```python
from build123d import *

# Parameters (mm, degrees)
F1_W          = 3
F1_H          = 12
F2_DEPTH      = 5
F2_DEPTH_BACK = 5
F4_R          = 3
F5_R          = 2.99999
F7_DEPTH      = 25
F8_R          = 3


# Not quite as in the source:
# - a fillet or chamfer is up to 0.001 mm smaller than in the source, because OpenCascade refuses the exact size


with BuildPart() as f2:
    # F1 (on Front) → F2 (new body, two sides)
    with BuildSketch(Plane.XZ) as f2_sk:
        with Locations((-19, -6)):
            Rectangle(F1_W, F1_H)
        Polygon((-20.5, 0), (-17.5, 0), (-17.5, 12), (-23.5, 12), (-23.5, -22), (-36.5, -22), (-36.5, -25), (-20.5, -25), (-20.5, -12), align=None)
    extrude(amount=F2_DEPTH)
    extrude(f2_sk.sketch, amount=-F2_DEPTH_BACK)

    # F0 (on Front) → F3 (revolve, cut)
    with BuildSketch(Plane.XZ):
        with BuildLine():
            Line((0, -20.5), (0, 20.5))
            ThreePointArc((0, 20.5), (-20.5, 0), (0, -20.5))
        make_face()
    revolve(axis=Axis((0, 0, 0), (0, 0, 1)), mode=Mode.SUBTRACT)

    # F4
    f4_edges = [f2.edges().sort_by_distance(p)[0] for p in [
        (-23.5, 0, 12),
        (-23.5, 0, -22),
    ]]
    fillet(f4_edges, radius=F4_R)

    # F5 (radius 3 in the source; OpenCascade refuses exactly that, so slightly less here)
    f5_edges = [f2.edges().sort_by_distance(p)[0] for p in [
        (-20.5, 0, -12),
    ]]
    fillet(f5_edges, radius=F5_R)

    # F6 (on face) → F7 (cut)
    with BuildSketch(Plane.XY.offset(-22)):
        with BuildLine():
            ThreePointArc((-29.75, 0), (-30.8303039934, 1.6167891819), (-32.7374368671, 1.2374368671))
            Line((-32.7374368671, 1.2374368671), (-30.2625631329, -1.2374368671))
            ThreePointArc((-30.2625631329, -1.2374368671), (-29.8832108181, -0.6696960066), (-29.75, 0))
        make_face()
        with BuildLine():
            Line((-30.2625631329, -1.2374368671), (-32.7374368671, 1.2374368671))
            ThreePointArc((-32.7374368671, 1.2374368671), (-32.7374368671, -1.2374368671), (-30.2625631329, -1.2374368671))
        make_face()
    extrude(amount=-F7_DEPTH, mode=Mode.SUBTRACT)

    # F8
    f8_edges = [f2.edges().sort_by_distance(p)[0] for p in [
        (-36.5, -5, -23.5),
        (-36.5, 5, -23.5),
    ]]
    fillet(f8_edges, radius=F8_R)


solid = f2.part
```
Verification items for the finished model (mm, model axes). A direction names the side the tool comes from. Coordinates: 2 decimals unless noted, no trailing zeros. Order: outer loops, then holes, each group sorted by start corner. A loop starts at its lowest first (then second) coordinate and runs counter-clockwise, first axis right, second up. Notation, with made-up numbers: (88.5, -25) -> (130.5, -25) arc R24 cw to (130.5, 13) -> close; hole circle Ø10 at (83, 12). An arc over 180 degrees is marked (long way). Put each result on its own line as item: value. Start each with the question number.
1) Tool access check on faces 1 (the flat face through (-20.5, 0, -20)), 2 (the flat face through (-23, 5, -8)), 3 (the flat face through (-29, 0, -22)). Record the directions out of +Z, -Z, +X, -X, +Y, -Y that give a thin tool (end or side, any length) a straight path to the whole face; none if there is none.
2) Cross-section at D-D (x = -27.75). Enter the section's corners in (y, z), plus the area to 3 significant figures.
3) Material ranges on L1, parallel to X at y = -1.5, z = -18; L2, parallel to Z at x = -33, y = 4; L3, parallel to Z at x = -24, y = -0.75, recorded low to high.
4) Cross-section at A-A (x = -31.5). Enter the section's corners in (y, z).
5) Cross-section at C-C (z = -18). Enter the section's corners in (x, y), plus the area to 3 significant figures.
6) Go/stop test with flat-tipped pins: pin 1 (5 mm diameter, centred on y = -1, z = -2.5, fed in from +X); pin 2 (4 mm diameter, centred on x = -26.5, y = 4, fed in from +Z); pin 3 (2 mm diameter, centred on y = 1, z = -15.5, fed in from +X). Record where each tip stops, or that it passes through.
Geometry check:
1. face 1: -Z, +X, +Y, -Y
1. face 2: +Z, -Z, +X, -X, +Y
1. face 3: +Z, -X, +Y, -Y
2. outline: (-5, -25) -> (5, -25) -> (5, -22) -> (-5, -22) -> close
2. area: 30.0 mm^2
3. L1: x = -23.5 to -20.5
3. L2: z = -25 to -22
3. L3: z = -25 to -20.66
4. outline: (-5, -25) -> (-1.75, -25) -> (-1.75, -22) -> (-5, -22) -> close; (1.75, -25) -> (5, -25) -> (5, -22) -> (1.75, -22) -> close
5. outline: (-23.5, -5) -> (-20.5, -5) -> (-20.5, 5) -> (-23.5, 5) -> close
5. area: 30.0 mm^2
6. pin 1: stops at x = -19.83
6. pin 2: stops at z = -21.24
6. pin 3: stops at x = -20.46
